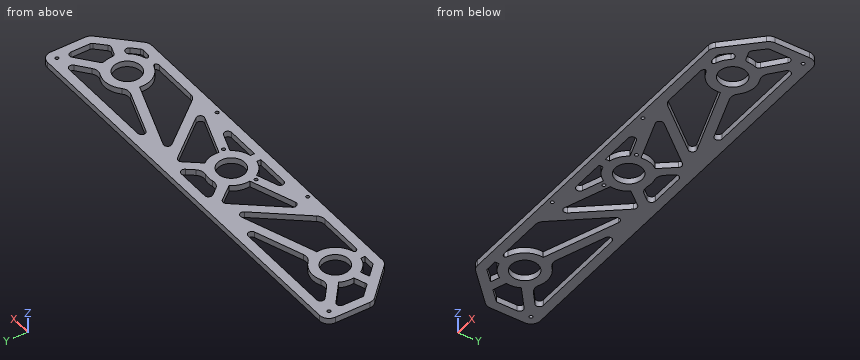
from build123d import *

# Parameters (mm, degrees)
SKETCH1_R           = 14.2875
BOSS_EXTRUDE1_DEPTH = 6.35
BOSS_EXTRUDE2_DEPTH = 6.35
FILLET1_R           = 10
FILLET2_R           = 4
FILLET3_R           = 4
SKETCH3_R           = 1.778
CUT_EXTRUDE1_DEPTH  = 10
SKETCH4_R           = 1.778
CUT_EXTRUDE2_DEPTH  = 10


with BuildPart() as part:
    # Sketch1 → Boss-Extrude1 (new body)
    with BuildSketch(Plane.XY):
        with BuildLine():
            Line((2.928932188, 35.171067812), (35.171067812, 2.928932188))
            ThreePointArc((35.171067812, 2.928932188), (38.4153013, 0.761204675), (42.242135624, 0))
            Line((42.242135624, 0), (402.257864376, 0))
            ThreePointArc((402.257864376, 0), (406.0846987, 0.761204675), (409.328932188, 2.928932188))
            Line((409.328932188, 2.928932188), (441.571067812, 35.171067812))
            ThreePointArc((441.571067812, 35.171067812), (443.738795325, 38.4153013), (444.5, 42.242135624))
            Line((444.5, 42.242135624), (444.5, 78.9))
            ThreePointArc((444.5, 78.9), (441.571067812, 85.971067812), (434.5, 88.9))
            Line((434.5, 88.9), (10, 88.9))
            ThreePointArc((10, 88.9), (2.928932188, 85.971067812), (0, 78.9))
            Line((0, 78.9), (0, 42.242135624))
            ThreePointArc((0, 42.242135624), (0.761204675, 38.4153013), (2.928932188, 35.171067812))
        make_face()
        with Locations((60, 38.1)):
            Circle(SKETCH1_R, mode=Mode.SUBTRACT)
        with Locations((384.5, 38.1)):
            Circle(SKETCH1_R, mode=Mode.SUBTRACT)
        with Locations((222.25, 38.1)):
            Circle(SKETCH1_R, mode=Mode.SUBTRACT)
        with BuildLine():
            Line((42.242135624, 10), (55, 10))
            Line((55, 10), (55, 14.332739824))
            ThreePointArc((55, 14.332739824), (45.977844894, 18.269169901), (39.258984185, 25.463033624))
            Line((39.258984185, 25.463033624), (30.039080729, 22.203054895))
            Line((30.039080729, 22.203054895), (42.242135624, 10))
        make_face(mode=Mode.SUBTRACT)
        with BuildLine():
            Line((402.257864376, 10), (414.460919271, 22.203054895))
            Line((414.460919271, 22.203054895), (405.241015815, 25.463033624))
            ThreePointArc((405.241015815, 25.463033624), (398.522155106, 18.269169901), (389.5, 14.332739824))
            Line((389.5, 14.332739824), (389.5, 10))
            Line((389.5, 10), (402.257864376, 10))
        make_face(mode=Mode.SUBTRACT)
        with BuildLine():
            Line((434.5, 42.242135624), (434.5, 72.446597797))
            Line((434.5, 72.446597797), (406.075642814, 49.252322333))
            ThreePointArc((406.075642814, 49.252322333), (408.427959025, 42.263584169), (408.574576932, 34.891043503))
            Line((408.574576932, 34.891043503), (420.045712746, 30.835072751))
            Line((420.045712746, 30.835072751), (422.296945105, 30.039080729))
            Line((422.296945105, 30.039080729), (434.5, 42.242135624))
        make_face(mode=Mode.SUBTRACT)
        with BuildLine():
            Line((17.908581132, 78.9), (159.303289572, 78.9))
            Line((159.303289572, 78.9), (80.698128287, 50.807090212))
            ThreePointArc((80.698128287, 50.807090212), (64.123087075, 62.034970424), (44.746603764, 57.000173532))
            Line((44.746603764, 57.000173532), (17.908581132, 78.9))
        make_face(mode=Mode.SUBTRACT)
        with BuildLine():
            Line((10, 42.242135624), (10, 72.446597797))
            Line((10, 72.446597797), (38.424357186, 49.252322333))
            ThreePointArc((38.424357186, 49.252322333), (36.072040975, 42.263584169), (35.925423068, 34.891043503))
            Line((35.925423068, 34.891043503), (24.454287254, 30.835072751))
            Line((24.454287254, 30.835072751), (22.203054895, 30.039080729))
            Line((22.203054895, 30.039080729), (10, 42.242135624))
        make_face(mode=Mode.SUBTRACT)
        with BuildLine():
            Line((65, 14.332739824), (65, 10))
            Line((65, 10), (128.768147223, 10))
            Line((128.768147223, 10), (141.942274838, 14.708336864))
            Line((141.942274838, 14.708336864), (198.186421388, 34.809583517))
            ThreePointArc((198.186421388, 34.809583517), (198.85545044, 44.625159549), (203.363262878, 53.370030031))
            Line((203.363262878, 53.370030031), (185.140287975, 75.742288539))
            Line((185.140287975, 75.742288539), (184.022239752, 77.114910957))
            Line((184.022239752, 77.114910957), (175.842867511, 74.191663136))
            Line((175.842867511, 74.191663136), (84.063578612, 41.390416483))
            ThreePointArc((84.063578612, 41.390416483), (79.854530137, 24.1114229), (65, 14.332739824))
        make_face(mode=Mode.SUBTRACT)
        with BuildLine():
            Line((399.753396236, 57.000173532), (426.591418868, 78.9))
            Line((426.591418868, 78.9), (285.196710428, 78.9))
            Line((285.196710428, 78.9), (363.801871713, 50.807090212))
            ThreePointArc((363.801871713, 50.807090212), (380.376912925, 62.034970424), (399.753396236, 57.000173532))
        make_face(mode=Mode.SUBTRACT)
        with BuildLine():
            Line((158.481852777, 10), (201.551871713, 25.392909788))
            ThreePointArc((201.551871713, 25.392909788), (208.2614229, 18.245469863), (217.25, 14.332739824))
            Line((217.25, 14.332739824), (217.25, 10))
            Line((217.25, 10), (158.481852777, 10))
        make_face(mode=Mode.SUBTRACT)
        with BuildLine():
            Line((195.465766991, 78.9), (211.116677179, 59.685452953))
            ThreePointArc((211.116677179, 59.685452953), (222.25, 62.3875), (233.383322821, 59.685452953))
            Line((233.383322821, 59.685452953), (249.034233009, 78.9))
            Line((249.034233009, 78.9), (195.465766991, 78.9))
        make_face(mode=Mode.SUBTRACT)
        with BuildLine():
            Line((379.5, 14.332739824), (379.5, 10))
            Line((379.5, 10), (315.731852777, 10))
            Line((315.731852777, 10), (302.557725162, 14.708336864))
            Line((302.557725162, 14.708336864), (246.313578612, 34.809583517))
            ThreePointArc((246.313578612, 34.809583517), (245.64454956, 44.625159549), (241.136737122, 53.370030031))
            Line((241.136737122, 53.370030031), (259.359712025, 75.742288539))
            Line((259.359712025, 75.742288539), (260.477760248, 77.114910957))
            Line((260.477760248, 77.114910957), (268.657132489, 74.191663136))
            Line((268.657132489, 74.191663136), (360.436421388, 41.390416483))
            ThreePointArc((360.436421388, 41.390416483), (364.645469863, 24.1114229), (379.5, 14.332739824))
        make_face(mode=Mode.SUBTRACT)
        with BuildLine():
            Line((286.018147223, 10), (227.25, 10))
            Line((227.25, 10), (227.25, 14.332739824))
            ThreePointArc((227.25, 14.332739824), (236.2385771, 18.245469863), (242.948128287, 25.392909788))
            Line((242.948128287, 25.392909788), (286.018147223, 10))
        make_face(mode=Mode.SUBTRACT)
    extrude(amount=BOSS_EXTRUDE1_DEPTH)

    # Sketch2 → Boss-Extrude2 (add)
    with BuildSketch(Plane.XY.offset(6.35)):
        Polygon((184.022239752, 77.114910957), (174.845752388, 73.835301483), (124.908015982, 13.177953241), (122.291683488, 10), (128.768147223, 10), (137.944634587, 13.279609474), (187.243188129, 73.160568149), align=None)
        Polygon((269.654247612, 73.835301483), (319.591984018, 13.177953241), (322.208316512, 10), (315.731852777, 10), (306.555365413, 13.279609474), (257.256811871, 73.160568149), (260.477760248, 77.114910957), align=None)
    extrude(amount=-BOSS_EXTRUDE2_DEPTH)

    # Fillet1
    fillet1_edges = [part.edges().sort_by_distance(p)[0] for p in [
        (211.116677179, 59.685452953, 3.175),
        (233.383322821, 59.685452953, 3.175),
        (44.746603764, 57.000173532, 3.175),
        (80.698128287, 50.807090212, 3.175),
        (399.753396236, 57.000173532, 3.175),
        (363.801871713, 50.807090212, 3.175),
        (122.291683488, 10, 3.175),
        (322.208316512, 10, 3.175),
    ]]
    fillet(fillet1_edges, radius=FILLET1_R)

    # Fillet2
    fillet2_edges = [part.edges().sort_by_distance(p)[0] for p in [
        (249.034233009, 78.9, 3.175),
        (195.465766991, 78.9, 3.175),
        (286.018147223, 10, 3.175),
        (159.303289572, 78.9, 3.175),
        (17.908581132, 78.9, 3.175),
        (158.481852777, 10, 3.175),
        (10, 72.446597797, 3.175),
        (426.591418868, 78.9, 3.175),
        (285.196710428, 78.9, 3.175),
        (434.5, 72.446597797, 3.175),
        (174.845752388, 73.835301483, 3.175),
        (187.243188129, 73.160568149, 3.175),
        (137.944634587, 13.279609474, 3.175),
        (269.654247612, 73.835301483, 3.175),
        (306.555365413, 13.279609474, 3.175),
        (257.256811871, 73.160568149, 3.175),
    ]]
    fillet(fillet2_edges, radius=FILLET2_R)

    # Fillet3
    # the kernel refuses this fillet: 4 mm, written as the material it adds along each edge
    with BuildSketch(Plane(origin=(434.5, 42.242135624, 0), x_dir=(0, 1, 0), z_dir=(0, 0, 1)), Plane(origin=(402.257864376, 10, 0), x_dir=(0.7071067811865684, 0.7071067811865266, 0), z_dir=(0, 0, 1))) as fillet3_piece_1:
        with BuildLine():
            CenterArc((FILLET3_R * 0.414213562373, FILLET3_R), FILLET3_R, 225, 45)
            Line((-FILLET3_R * 0.292893218813, FILLET3_R * 0.292893218813), (0, 0))
            Line((0, 0), (FILLET3_R * 0.414213562373, 0))
        make_face()
    extrude(amount=6.35)
    with BuildSketch(Plane(origin=(422.296945105, 30.039080729, 0), x_dir=(-0.9428009879202438, 0.33335611165330736, 0), z_dir=(0, 0, 1))) as fillet3_piece_2:
        with BuildLine():
            CenterArc((FILLET3_R * 0.630618821441, -FILLET3_R), FILLET3_R, 90, 64.47260491)
            Line((-FILLET3_R * 0.271760517527, -FILLET3_R * 0.569057395232), (0, 0))
            Line((0, 0), (FILLET3_R * 0.630618821441, 0))
        make_face()
    extrude(amount=6.35)
    with BuildSketch(Plane(origin=(408.574576932, 34.891043503, 0), x_dir=(0.07422292500138471, 0.9972416745223992, 0), z_dir=(0, 0, 1)), Plane(origin=(389.5, 14.332739824, 0), x_dir=(0.9649431016089534, 0.262459159979783, 0), z_dir=(0, 0, 1)), Plane(origin=(65, 14.332739824, 0), x_dir=(0.9649431016089596, 0.2624591599797595, 0), z_dir=(0, 0, 1))) as fillet3_piece_3:
        with BuildLine():
            CenterArc((3.059187738, -3.993222777), FILLET3_R, 93.335760439, 71.44820939)
            Line((-0.800584668, -2.943386137), (0, 0))
            ThreePointArc((0, 0), (1.413219633, -0.04115045), (2.826439265, 0))
        make_face()
    extrude(amount=6.35)
    with BuildSketch(Plane(origin=(406.075642814, 49.252322333, 0), x_dir=(0.774785119901029, 0.632224657839243, 0), z_dir=(0, 0, 1))) as fillet3_piece_4:
        with BuildLine():
            CenterArc((3.050320928, -4), FILLET3_R, 90, 71.44820939)
            ThreePointArc((-0.741824875, -2.727353071), (-0.331204595, -1.374476848), (0, 0))
            Line((0, 0), (3.050320928, 0))
        make_face()
    extrude(amount=6.35)
    with BuildSketch(Plane(origin=(414.460919271, 22.203054895, 0), x_dir=(-0.9428009879202406, 0.33335611165331624, 0), z_dir=(0, 0, 1))) as fillet3_piece_5:
        with BuildLine():
            CenterArc((FILLET3_R * 1.58574398036, FILLET3_R), FILLET3_R, 154.47260491, 115.52739509)
            Line((FILLET3_R * 0.68336464139, FILLET3_R * 1.43094260477), (0, 0))
            Line((0, 0), (FILLET3_R * 1.58574398036, 0))
        make_face()
    extrude(amount=6.35)
    with BuildSketch(Plane(origin=(405.241015815, 25.463033624, 0), x_dir=(-0.5691164356367163, -0.82225694444508, 0), z_dir=(0, 0, 1)), Plane(origin=(379.5, 14.332739824, 0), x_dir=(-0.9649431016089597, 0.2624591599797589, 0), z_dir=(0, 0, 1))) as fillet3_piece_6:
        with BuildLine():
            CenterArc((3.059187738, 3.993222777), FILLET3_R, 195.216030171, 71.44820939)
            Line((-0.800584668, 2.943386137), (0, 0))
            ThreePointArc((0, 0), (1.413219633, 0.04115045), (2.826439265, 0))
        make_face()
    extrude(amount=6.35)
    with BuildSketch(Plane(origin=(389.5, 10, 0), x_dir=(1, 0, 0), z_dir=(0, 0, 1)), Plane(origin=(65, 10, 0), x_dir=(1, 0, 0), z_dir=(0, 0, 1))) as fillet3_piece_7:
        with BuildLine():
            CenterArc((FILLET3_R, FILLET3_R), FILLET3_R, 180, 90)
            Line((0, FILLET3_R), (0, 0))
            Line((0, 0), (FILLET3_R, 0))
        make_face()
    extrude(amount=6.35)
    with BuildSketch(Plane(origin=(379.5, 10, 0), x_dir=(-1, 0, 0), z_dir=(0, 0, 1))) as fillet3_piece_8:
        with BuildLine():
            CenterArc((FILLET3_R, -FILLET3_R), FILLET3_R, 90, 90)
            Line((0, -FILLET3_R), (0, 0))
            Line((0, 0), (FILLET3_R, 0))
        make_face()
    extrude(amount=6.35)

    # Sketch3 → Cut-Extrude1 (cut)
    with BuildSketch(Plane(origin=(0, 0, 0), x_dir=(-1, 0, 0), z_dir=(0, 0, -1))):
        with Locations((-434.5, 78.9)):
            Circle(SKETCH3_R)
        with Locations((-247.620647359, 29.032716175)):
            Circle(SKETCH3_R)
        with Locations((-196.879352641, 29.032716175)):
            Circle(SKETCH3_R)
        with Locations(Location((-10, 78.9, 0), (0, 0, 180))):
            Circle(SKETCH3_R)
    extrude(amount=-CUT_EXTRUDE1_DEPTH, mode=Mode.SUBTRACT)

    # Sketch4 → Cut-Extrude2 (cut)
    with BuildSketch(Plane(origin=(0, 0, 0), x_dir=(-1, 0, 0), z_dir=(0, 0, -1))):
        with Locations((-292.912963738, 5)):
            Circle(SKETCH4_R)
        with Locations((-151.587036262, 5)):
            Circle(SKETCH4_R)
    extrude(amount=-CUT_EXTRUDE2_DEPTH, mode=Mode.SUBTRACT)


solid = part.part
The model under review builds one solid part; all positions refer to its coordinate system, in mm. Round coordinates to 2 decimals unless told otherwise and drop trailing zeros. Loops run counter-clockwise (first coordinate to the right, second up) from the corner with the lowest first, then second, coordinate; pieces in that order, holes last. Notation, with made-up numbers: M 41,18.5 L 51,18.5 A25 cw 51,35.5 Z; hole C 21.5,84 d5. An arc over 180 degrees is marked long. Answer as a JSON object with one key per item and string values.
Item 1: We need section A-A, the plane x = 60. State the section outline as (y, z) points.
Check sheet entries:
{"outline": "M 0,0 L 23.81,0 L 23.81,6.35 L 0,6.35 Z; M 52.39,0 L 62.39,0 L 62.39,6.35 L 52.39,6.35 Z; M 78.9,0 L 88.9,0 L 88.9,6.35 L 78.9,6.35 Z"}
Item 2: Clearance check with flat-ended pins moving along their axes: P1, Ø17, axis at x = 384.5, y = 38.1, coming from the +Z side; P2, Ø10, axis at x = 307, y = 70.5, coming from the -Z side; P3, Ø1.3, axis at y = 13, z = 4, coming from the +X side. State where each tip first meets the part, or that it passes through.
Check sheet entries:
{"P1": "through", "P2": "z = 0", "P3": "x = 420.05"}
Item 3: We need section C-C, the plane x = 345. State the section outline as (y, z) points.
Check sheet entries:
{"outline": "M 0,0 L 10,0 L 10,6.35 L 0,6.35 Z; M 46.91,0 L 57.53,0 L 57.53,6.35 L 46.91,6.35 Z; M 78.9,0 L 88.9,0 L 88.9,6.35 L 78.9,6.35 Z"}
Item 4: We need section B-B, the plane z = 3.5. State how many separate pieces and enclosed holes the cut face has, and give its area (3 significant figures).
Check sheet entries:
{"separate pieces": "1", "enclosed holes": "22", "area": "20,500 mm2"}
Item 5: For line 1 along Y through (x, z) = (385, 4.5); line 2 along Y through (x, z) = (254, 6); line 3 along X through (y, z) = (74, 4), list the stretches that pass through material, from the lowest coordinate up.
Check sheet entries:
{"line 1": "0 to 23.82, 52.38 to 62.38, 78.9 to 88.9", "line 2": "0 to 10, 21.44 to 32.06, 69.16 to 88.9", "line 3": "0 to 25.24, 140.12 to 199.99, 244.51 to 304.38, 419.26 to 444.5"}
